```python
from build123d import *

# Parameters (mm, degrees)
F0_W     = 244
F0_H     = 25
F1_DEPTH = 12
F2_W     = 50
F2_H     = 25
F3_DEPTH = 40
F4_R     = 6.35
F5_DEPTH = 25.001
F6_R     = 20
F7_R     = 20
F8_R     = 3
F9_DEPTH = 52.001


with BuildPart() as f1:
    # F0 (on Front) → F1 (new body)
    with BuildSketch(Plane.XZ):
        with Locations((14.424432, -12.022949)):
            Rectangle(F0_W, F0_H)
    extrude(amount=F1_DEPTH)

    # F2 (on face) → F3 (join)
    with BuildSketch(Plane.XZ.offset(12)):
        with Locations((14.424432, -12.022949)):
            Rectangle(F2_W, F2_H)
    extrude(amount=F3_DEPTH)

    # F4 (on face) → F5 (cut, through all)
    with BuildSketch(Plane.XY.offset(0.477051)):
        with Locations((14.424432, -32)):
            Circle(F4_R)
    extrude(amount=-F5_DEPTH, mode=Mode.SUBTRACT)

    # F6
    f6_edges = [f1.edges().sort_by_distance(p)[0] for p in [
        (-10.575568, -52, -12.022949),
    ]]
    fillet(f6_edges, radius=F6_R)

    # F7
    f7_edges = [f1.edges().sort_by_distance(p)[0] for p in [
        (39.424432, -52, -12.022949),
    ]]
    fillet(f7_edges, radius=F7_R)

    # F8 (on face) → F9 (cut, through all)
    with BuildSketch(Plane(origin=(0, 0, 0), x_dir=(-1, 0, 0), z_dir=(0, 1, 0))):
        with Locations((87.575568, -12.022949)):
            Circle(F8_R)
        with Locations((57.575568, -12.022949)):
            Circle(F8_R)
        with Locations((-86.424432, -12.022949)):
            Circle(F8_R)
        with Locations((-116.424432, -12.022949)):
            Circle(F8_R)
        with Locations((-56.424432, -12.022949)):
            Circle(F8_R)
        with Locations((27.575568, -12.022949)):
            Circle(F8_R)
    extrude(amount=-F9_DEPTH, mode=Mode.SUBTRACT)


solid = f1.part
```
Can you work these out from the model? Positions are in its coordinate system, mm. A direction names the side the tool comes from. Round coordinates to 2 decimals unless told otherwise and drop trailing zeros. Loops run counter-clockwise (first coordinate to the right, second up) from the corner with the lowest first, then second, coordinate; pieces in that order, holes last. Notation, with made-up numbers: M 1.5,26.5 L 46.5,26.5 A22 cw 46.5,62.5 Z; hole C 82,24 d4. An arc over 180 degrees is marked long. Answer in a Markdown table with one row per item.
1. Please list where these lines run through material, in increasing order: line 1 (Y direction, x = -90, z = -9); line 2 (X direction, y = -37, z = -3.25); line 3 (X direction, y = -27, z = -6.25). Write a range as from..to.
Established:
| item | result |
|---|---|
| line 1 | -12..0 |
| line 2 | -9.94..10.51, 18.34..38.79 |
| line 3 | -10.58..10.51, 18.34..39.42 |
2. If we section it at A-A, the plane z = -2.5: Please give me the cut outline in (x, y), plus the area to 3 significant figures.
Established:
| item | result |
|---|---|
| outline | M -107.58,-12 L -10.58,-12 L -10.58,-32 A20 ccw 9.42,-52 L 19.42,-52 A20 ccw 39.42,-32 L 39.42,-12 L 136.42,-12 L 136.42,0 L -107.58,0 Z; hole C 14.42,-32 d12.7 |
| area | 4,630 mm² |
3. On a 3-axis mill with a long thin cutter (end or side, diameter ignored), from which of +Z, -Z, +X, -X, +Y, -Y can I reach the whole of each face in a straight line? I mean faces 4 (the face through (-60, -12, -9)), 5 (the face through (14, -16, 0.477)), 6 (the face through (39.424, -22, -12)). Say none if no direction works.
Established:
| item | result |
|---|---|
| face 4 | +Z, -Z, -X, -Y |
| face 5 | +Z, +X, -X, +Y, -Y |
| face 6 | +Z, -Z, +X, -Y |
4. If we section it at B-B, the plane x = 87: Please give me the cut outline in (y, z), plus the area to 3 significant figures.
Established:
| item | result |
|---|---|
| outline | M -12,-24.52 L 0,-24.52 L 0,-14.97 L -12,-14.97 Z; M -12,-9.08 L 0,-9.08 L 0,0.48 L -12,0.48 Z |
| area | 229 mm² |
5. If we section it at D-D, the plane y = -17: Please give me the cut outline in (x, z).
Established:
| item | result |
|---|---|
| outline | M -10.58,-24.52 L 39.42,-24.52 L 39.42,0.48 L -10.58,0.48 Z |
6. If we section it at C-C, the plane y = -4.5: Please give me the cut outline in (x, z), plus the area to 3 significant figures.
Established:
| item | result |
|---|---|
| outline | M -107.58,-24.52 L 136.42,-24.52 L 136.42,0.48 L -107.58,0.48 Z; hole C -87.58,-12.02 d6; hole C -57.58,-12.02 d6; hole C -27.58,-12.02 d6; hole C 56.42,-12.02 d6; hole C 86.42,-12.02 d6; hole C 116.42,-12.02 d6 |
| area | 5,930 mm² |
7. I'm going to push flat-ended pins straight in: pin 1 Ø3 at (y, z) = (-33, -6) entering from -X; pin 2 Ø7.5 at (x, z) = (88.5, -17) entering from -Y; pin 3 Ø10 at (y, z) = (-24, -12) entering from +X. Where does each tip first touch, or does it pass through?
Established:
| item | result |
|---|---|
| pin 1 | x = -10.58 |
| pin 2 | y = -12 |
| pin 3 | x = 39.42 |
8. Thinking about a two-plate mould opening in X: for faces 1 (the face through (-25.195, -5.916, -13.848)), 2 (the face through (-107.576, -6, -12)), 3 (the face through (13, 0, -12)), which applies, pulls with the +X half, pulls with the -X half, needs draft (parallel to the pull), parting line crosses it, or undercut?
Established:
| item | result |
|---|---|
| face 1 | undercut |
| face 2 | pulls with the -X half |
| face 3 | needs draft |
